Here's how the part is built. I have some questions about the finished solid (model axes, mm). Face numbers are marked on the shaded views. A direction names the side the tool comes from. Coordinates: 2 decimals unless noted, no trailing zeros. Loops run counter-clockwise (first coordinate to the right, second up) from the corner with the lowest first, then second, coordinate; pieces in that order, holes last. Notation, with made-up numbers: M 82.5,70.25 L 131.5,70.25 A18 cw 131.5,96.25 Z; hole C 67,82.5 d5. An arc over 180 degrees is marked long. Use one line per item in the form item = value. Start each with the question number.
(1) Please list where these lines run through material, in increasing order: L1, parallel to Y at x = 1, z = -0.05; L2, parallel to Y at x = -1.5, z = -2.45.
(2) Imagine slicing it at B-B, the plane x = 6.25. Please give me the cut outline in (y, z).
(3) Imagine slicing it at A-A, the plane x = -2. Please give me the cut outline in (y, z), and give its area (3 significant figures).
(4) Will these pins go through, and if not, where does the flat tip stop? P1, Ø1.5, axis at x = 2.5, y = 1.5, coming from the -Z side; P2, Ø2, axis at x = 5.5, y = -2, coming from the +Z side; P3, Ø0.7, axis at x = -1.5, y = -0.5, coming from the +Z side.
(5) Thinking about a two-plate mould opening in Y: for the marked faces 4, 5 and 6, which applies, +Y half, -Y half, draft (parallel to the pull), parting line (faces both ways), or undercut?
(6) On a 3-axis mill with a long thin cutter (end or side, diameter ignored), from which of +Z, -Z, +X, -X, +Y, -Y can I reach the whole of each face in a straight line? I mean the marked faces 1, 2 and 3. Say none if no direction works.
```python
from build123d import *

# Parameters (mm, degrees)
CUT_EXTRUDE1_DEPTH = 2.6


with BuildPart() as part:
    # Sketch1 → Revolve1 (revolve)
    with BuildSketch(Plane.XY, mode=Mode.PRIVATE) as revolve1_sk:
        with BuildLine():
            Line((-0.428312164, 0), (-1.15, 1.25))
            Line((-1.15, 1.25), (-3, 1.25))
            Line((-3, 1.25), (-3, 2.45))
            ThreePointArc((-3, 2.45), (-2.912132034, 2.662132034), (-2.7, 2.75))
            Line((-2.7, 2.75), (0, 2.75))
            Line((0, 2.75), (0, 1.8))
            ThreePointArc((0, 1.8), (0.015193643, 1.74701055), (0.056157637, 1.710123155))
            Line((0.056157637, 1.710123155), (0.466157637, 1.510123155))
            ThreePointArc((0.466157637, 1.510123155), (0.48750205, 1.50256365), (0.51, 1.5))
            Line((0.51, 1.5), (7.6935, 1.5))
            Line((7.6935, 1.5), (8, 1.1935))
            Line((8, 1.1935), (8, 0))
            Line((8, 0), (-0.428312164, 0))
        make_face()
    revolve(revolve1_sk.sketch.rotate(Axis((8, 0, 0), (-1, 0, 0)), 270), axis=Axis((8, 0, 0), (-1, 0, 0)))

    # Sketch2 → Cut-Extrude1 (cut)
    with BuildSketch(Plane(origin=(-1.15, 0, 0), x_dir=(0, 0, -1), z_dir=(1, 0, 0))):
        Polygon((-1.25, 0.721687836), (-1.25, -0.721687836), (0, -1.443375673), (1.25, -0.721687836), (1.25, 0.721687836), (0, 1.443375673), align=None)
    extrude(amount=-CUT_EXTRUDE1_DEPTH, mode=Mode.SUBTRACT)


solid = part.part
```
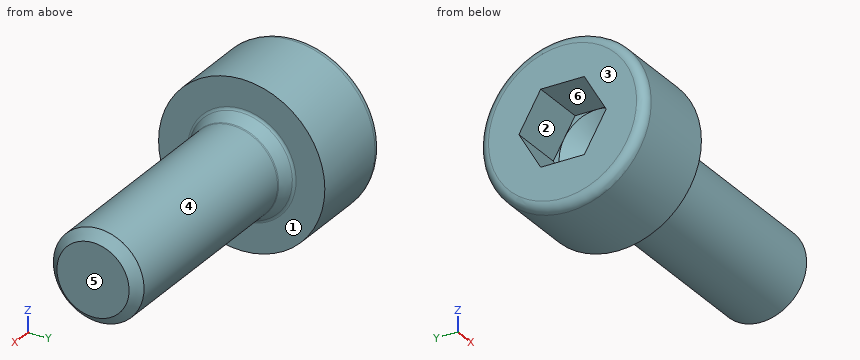
Answer:
q1.L1 = -1.5 to 1.5
q1.L2 = -1.25 to 1.25
q2.outline = C 0,0 d3
q3.outline = C 0,0 d5.5; hole M -1.44,0 L -0.72,-1.25 L 0.72,-1.25 L 1.44,0 L 0.72,1.25 L -0.72,1.25 Z
q3.area = 18.3 mm²
q4.P1 = -1.3
q4.P2 = 1.12
q4.P3 = 2.75
q5.face_4 = parting line
q5.face_5 = draft
q5.face_6 = undercut
q6.face_1 = +X
q6.face_2 = -X
q6.face_3 = +Z, -Z, -X, +Y, -Y
